Geometry: final body of the model. Coordinates: model frame, mm. A direction names the side the tool comes from. Coordinates: 2 decimals unless noted, no trailing zeros. Write each loop counter-clockwise with the first axis right and the second up, starting at its lowest first coordinate (ties: lowest second). Pieces come first, ordered by that corner, then holes. Notation, with made-up numbers: (-32, 29) -> (26, 29) arc R24 ccw to (26, 48) -> close; hole circle Ø10 at (-12.75, 4.5). An arc over 180 degrees is marked (long way). One line per item, written item: value.
```python
from build123d import *

# Parameters (mm, degrees)
F0_R         = 3.9
F2_DEPTH     = 14
F3_R         = 7.5
F4_DEPTH     = 5
F6_R         = 4.3
F7_DEPTH     = 4.1
F1_R         = 1.5693660879
F8_DEPTH     = 23.4
F9_DEPTH     = 15.5
F10_R        = 0.2
F11_S5_R     = 4.3
F11_T6_DEPTH = 9
F12_R        = 1.5
F13_R        = 1.5


# Not quite as in the source:
# - a fillet or chamfer that OpenCascade refuses, or shapes differently, is made with other operations: its cross-section is extruded or revolved along the edge and cut away or added


with BuildPart() as f2:
    # F0 (on Top) → F2 (new body)
    with BuildSketch(Plane.XY):
        with Locations((-41.4718948305, -26.0946750641)):
            Circle(F0_R)
    extrude(amount=F2_DEPTH)

    # F3 (on face) → F4 (join)
    with BuildSketch(Plane.XY.offset(14)):
        with Locations((-41.4718948305, -26.0946750641)):
            Circle(F3_R)
    extrude(amount=F4_DEPTH)

    # F6 (on face) → F7 (join)
    with BuildSketch(Plane(origin=(0, 0, 14), x_dir=(1, 0, 0), z_dir=(0, 0, -1))):
        with Locations((-41.4718948305, 26.0946750641)):
            Circle(F6_R)
    extrude(amount=F7_DEPTH)

    # F1 (on Top) → F8 (cut)
    with BuildSketch(Plane.XY):
        with Locations((-41.495975107, -26.0728988796)):
            Circle(F1_R)
    extrude(amount=F8_DEPTH, mode=Mode.SUBTRACT)

    # F5 (on face) → F9 (cut)
    with BuildSketch(Plane.XY.offset(19)):
        Polygon((-39.9783341683, -29.0917753096), (-38.1295495491, -26.2997637113), (-39.6231102113, -23.3026634658), (-42.9654554927, -23.0975748186), (-44.8142401119, -25.8895864169), (-43.3206794497, -28.8866866624), align=None)
    extrude(amount=-F9_DEPTH, mode=Mode.SUBTRACT)

    # F10
    f10_edges = [f2.edges().sort_by_distance(p)[0] for p in [
        (-45.371895, -26.094675, 0),
    ]]
    fillet(f10_edges, radius=F10_R)

    # F11: chamfer of 8 x 0.4612770977 on 1 edges, made by hand


with BuildPart() as f11_tool2:
    # F11_s3 → F11_t4 (revolve)
    with BuildSketch(Plane.XZ.offset(26.0946750641)):
        Polygon((-37.5718948305, 1.9), (-37.1106177328, 9.9), (-37.5718948305, 9.9), align=None)
    revolve(axis=Axis((-41.4718948305, -26.0946750641, 9.9), (0, 0, -1)))

    # F11_s5 → F11_t6 (intersect, symmetric)
    with BuildSketch(Plane.XY.offset(5.9)):
        with Locations((-41.4718948305, -26.0946750641)):
            Circle(F11_S5_R)
    extrude(amount=F11_T6_DEPTH, both=True, mode=Mode.INTERSECT)


with BuildPart() as f2_1:
    add(f2.part)

    # F11_t1: union F11_tool2
    add(f11_tool2.part)

    # F12
    f12_edges = [f2_1.edges().sort_by_distance(p)[0] for p in [
        (-48.971895, -26.094675, 14),
    ]]
    fillet(f12_edges, radius=F12_R)

    # F13
    f13_edges = [f2_1.edges().sort_by_distance(p)[0] for p in [
        (-48.971895, -26.094675, 19),
    ]]
    fillet(f13_edges, radius=F13_R)


solid = f2_1.part
```
(1) First-contact query: pin 1 (1.8 mm diameter, centred on x = -43, y = -25, fed in from +Z); pin 2 (3 mm diameter, centred on y = -30.5, z = 7, fed in from -X). Flat tips, straight axial feed; report the tip coordinate or a pass-through.
Responses:
pin 1: stops at z = 3.5
pin 2: stops at x = -44.5
(2) Pull-direction query (Y, two-part tool) for faces 4 (the flat face through (-42, -28, 0)), 5 (the flat face through (-40, -27, 3.5)), 6 (the cylindrical face through (-41.98, -22.228, 1.038)), 7 (the flat face through (-41.3, -23.2, 11.4)); classes: released by +Y, released by -Y, zero draft, split by the parting line, or undercut.
Responses:
face 4: zero draft
face 5: undercut
face 6: split by the parting line
face 7: undercut
(3) Reachability of faces 1 (the flat face through (-46, -25, 14)), 2 (the flat face through (-39.07, -27.72, 11.36)), 3 (the cylindrical face through (-38.01, -32.75, 16.49)) from +Z, -Z, +X, -X, +Y, -Y: full face, straight path, thin tool, end or side. Return the list, or none.
Responses:
face 1: -Z
face 2: +Z
face 3: +Z, -Z
(4) Section B-B (z = 7.75). Return the cut outline in (x, y), then the cut area to 3 significant figures.
Responses:
outline: circle Ø8.47 at (-41.47, -26.09); hole (-44.81, -25.89) -> (-43.32, -28.89) -> (-39.98, -29.09) -> (-38.13, -26.3) -> (-39.62, -23.3) -> (-42.97, -23.1) -> close
area: 27.3 mm2
(5) Line query: line 1 (Y direction, x = -42.5, z = 9); line 2 (Z direction, x = -38, y = -29.25); line 3 (Y direction, x = -38.25, z = 17). Output: solid intervals per line, ascending. Write a range as [from, to].
Responses:
line 1: y = [-30.27, -28.94], [-23.13, -21.92]
line 2: z = [14, 19]
line 3: y = [-32.87, -26.48], [-26.06, -19.32]
(6) Section C-C (z = 2.5). Return the cut outline in (x, y).
Responses:
outline: circle Ø7.87 at (-41.47, -26.09); hole circle Ø3.14 at (-41.5, -26.07)
(7) Section A-A (z = 12.5). Return the cut outline in (x, y), then the cut area to 3 significant figures.
Responses:
outline: circle Ø8.6 at (-41.47, -26.09); hole (-44.81, -25.89) -> (-43.32, -28.89) -> (-39.98, -29.09) -> (-38.13, -26.3) -> (-39.62, -23.3) -> (-42.97, -23.1) -> close
area: 29.0 mm2
